The listing builds one solid part. Answer for the finished solid, in the listing's coordinates (mm). A direction names the side the tool comes from. Give positions to 0.01 mm unless a question says otherwise; leave off trailing zeros. Write each loop counter-clockwise with the first axis right and the second up, starting at its lowest first coordinate (ties: lowest second). Pieces come first, ordered by that corner, then holes. Notation, with made-up numbers: (-38, -13) - (-7, -13) arc R16 ccw to (-7, 14) - close; hole circle Ø7 at (39.5, 56.25). An arc over 180 degrees is marked (long way). Return JSON: item names as keys, results as strings.
Autodesk Inventor part; units mm, degrees
ref_plane "YZ Plane" through (0, 0, 0) normal (1, 0, 0) x (0, 1, 0)
ref_plane "XZ Plane" through (0, 0, 0) normal (0, 1, 0) x (-1, 0, 0)
ref_plane "XY Plane" through (0, 0, 0) normal (0, 0, 1) x (1, 0, 0)
sketch "Skizze1" plane through (0, 0, 0) normal (0, 0, 1) x (1, 0, 0)
  line L0 (-0.75, 28.5) -> (0, 28.5)
  line L1 (-3.3, 20) -> (-2, 20)
  line L2 (-2, 15) -> (-0.75, 15)
  line L3 (0, 28.5) -> (0, 0)
  line L4 (-0.75, 0) -> (-0.75, 15)
  line L5 (-2, 15) -> (-2, 20)
  line L6 (-3.3, 20) -> (-3.3, 22)
  line L7 (-0.75, 28.5) -> (-0.75, 22)
  line L8 (-0.75, 0) -> (0, 0)
  line L9 (-3.96, 0) -> (0.66, 0)
  line L10 (0, -5.7) -> (0, 34.2)
  line L11 (-0.75, 22) -> (-3.3, 22)
  point P0 (0, 0)
  dimension "d0" = 1.5
  dimension "d1" = 4
  dimension "d2" = 6.6
  dimension "d3" = 1.5
  dimension "d5" = 5
  dimension "d6" = 15
  dimension "d9" = 6.5
  dimension "d10" = 2
revolve "Umdrehung1" add sketch "Skizze1" angle 360 about axis through (0, -10, 0) along (0, 1, 0)
fillet "Rundung1" radius 0.2 3 edges at (0.75, 15, 0) (2, 20, 0) (0.75, 22, 0)
chamfer "Fase1" distance 0.2 angle 45 5 edges at (0.75, 0, 0) (2, 15, 0) (3.3, 20, 0) (3.3, 22, 0) (0.75, 28.5, 0)
properties part number "YTP-AP-E17-R1.0"
Item 1: Consider L1, parallel to Y at x = -1.5, z = 0.25; L2, parallel to Y at x = 2.5, z = 1; L3, parallel to X at y = 14, z = -0.5. Determine where each line is inside the solid, lowest interval first.
Answer below:
{"L1": "y = 15 to 22", "L2": "y = 20 to 22", "L3": "x = -0.56 to 0.56"}
Item 2: A cutting plane is placed at C-C on y = 25. Determine the outline of the cut face in (x, z).
Answer below:
{"outline": "circle Ø1.5 at (0, 0)"}
Item 3: Flat-ended cylindrical pins translate along their axes: P1, Ø1.5, axis at y = 24, z = -2, coming from the -X side; P2, Ø3, axis at x = -1, z = -2.5, coming from the +Y side; P3, Ø2, axis at x = 2.5, z = 2.5, coming from the -Y side. Find the tip coordinate at first contact, or state that the pin passes through.
Answer below:
{"P1": "passes through", "P2": "stops at y = 22", "P3": "stops at y = 20"}
Item 4: For faces 1 (the face through (0.75, 7.6, 0.03)), 2 (the face through (0, 28.5, 0)), 3 (the face through (-1, 22, 1)), determine the directions among +Z, -Z, +X, -X, +Y, -Y from which every point of the face is accessible in a straight line to the end or side of a thin tool.
Answer below:
{"face 1": "-Y", "face 2": "+Z, -Z, +X, -X, +Y", "face 3": "+Y"}
